Read the model definition and answer for the solid it produces. Units are mm, in the model's axes. Round coordinates to 2 decimals unless told otherwise and drop trailing zeros. Order: outer loops, then holes, each group sorted by start corner. A loop starts at its lowest first (then second) coordinate and runs counter-clockwise, first axis right, second up. Notation, with made-up numbers: (2.25, -39) - (13.25, -39) arc R15 ccw to (13.25, -34) - close; hole circle Ø1 at (80, -31.75). An arc over 180 degrees is marked (long way). Put each result on its own line as item: value. Start each with the question number.
Q1. Section C-C on z = 2.5 is taken. Give the vertices of the cut face in (x, y).
Q2. Each of these flat-tipped pins is pushed along its axis until it touches: pin 1 Ø1.2 at (x, z) = (12, 3) entering from -Y; pin 2 Ø1 at (y, z) = (12, 3) entering from -X; pin 3 Ø0.6 at (y, z) = (22.5, 3) entering from +X; pin 4 Ø1.2 at (x, y) = (-1.5, 10) entering from +Z. Where does it stop, or does it pass through?
Q3. Section B-B on y = 16 is taken. Give the vertices of the cut face in (x, z).
Q4. Section A-A on x = 12 is taken. Give the vertices of the cut face in (y, z).
Q5. Section D-D on y = 32 is taken. Give the vertices of the cut face in (x, z).
Q6. Find the intervals of material crossed by line 1 along Y through (x, z) = (12, 2.2); line 2 along X through (y, z) = (18, 1.4); line 3 along X through (y, z) = (29.5, 1.45), in increasing order. Write a range as from..to.
from build123d import *

# Parameters (mm, degrees)
SKETCH_W     = 42
SKETCH_H     = 35
SKETCH_R     = 10
PAD_DEPTH    = 4
SKETCH001_W  = 2.5
SKETCH001_H  = 6
POCKET_DEPTH = 5
SKETCH002_W  = 35
SKETCH002_H  = 2
PAD001_DEPTH = 2.5
SKETCH003_W  = 35
SKETCH003_H  = 2
PAD002_DEPTH = 2.5


with BuildPart() as part:
    # Sketch → Pad (new body)
    with BuildSketch(Plane.XY):
        with Locations((21, 17.5)):
            Rectangle(SKETCH_W, SKETCH_H)
        with Locations((12, 18)):
            Circle(SKETCH_R, mode=Mode.SUBTRACT)
    extrude(amount=PAD_DEPTH)

    # Sketch001 (on Face7 of Pad) → Pocket (cut)
    with BuildSketch(Plane.XY.offset(4)):
        with Locations((12, 27.5)):
            Rectangle(SKETCH001_W, SKETCH001_H)
    extrude(amount=-POCKET_DEPTH, mode=Mode.SUBTRACT)

    # Sketch002 (on Face3 of Pocket) → Pad001 (join)
    with BuildSketch(Plane.YZ.offset(42)):
        with Locations((17.5, 1)):
            Rectangle(SKETCH002_W, SKETCH002_H)
    extrude(amount=PAD001_DEPTH)

    # Sketch003 (on Face2 of Pad001) → Pad002 (join)
    with BuildSketch(Plane(origin=(0, 0, 0), x_dir=(0, -1, 0), z_dir=(-1, 0, 0))):
        with Locations((-17.5, 1)):
            Rectangle(SKETCH003_W, SKETCH003_H)
    extrude(amount=PAD002_DEPTH)


solid = part.part
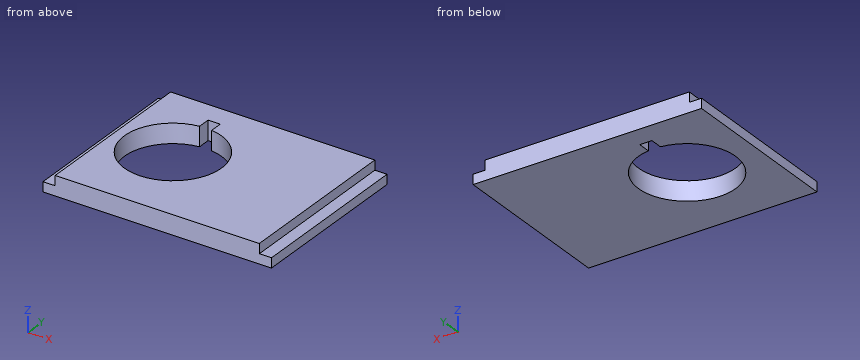
Findings:
1. outline: (0, 0) - (42, 0) - (42, 35) - (0, 35) - close; hole (10.75, 27.92) arc R10 ccw (long way) to (13.25, 27.92) - (13.25, 30.5) - (10.75, 30.5) - close
2. pin 1: y = 0
2. pin 2: x = 0
2. pin 3: x = 42
2. pin 4: z = 2
3. outline: (-2.5, 0) - (2.2, 0) - (2.2, 4) - (0, 4) - (0, 2) - (-2.5, 2) - close; (21.8, 0) - (44.5, 0) - (44.5, 2) - (42, 2) - (42, 4) - (21.8, 4) - close
4. outline: (0, 0) - (8, 0) - (8, 4) - (0, 4) - close; (30.5, 0) - (35, 0) - (35, 4) - (30.5, 4) - close
5. outline: (-2.5, 0) - (44.5, 0) - (44.5, 2) - (42, 2) - (42, 4) - (0, 4) - (0, 2) - (-2.5, 2) - close
6. line 1: 0..8, 30.5..35
6. line 2: -2.5..2, 22..44.5
6. line 3: -2.5..10.75, 13.25..44.5
